For this review, use the dimensioned drawing (mm, ordinates from the lowest corner) and the shaded views. A direction names the side the tool comes from. Round coordinates to 2 decimals unless told otherwise and drop trailing zeros. Loops run counter-clockwise (first coordinate to the right, second up) from the corner with the lowest first, then second, coordinate; pieces in that order, holes last. Notation, with made-up numbers: (43.25, -31) - (65.25, -31) arc R25 cw to (65.25, 3) - close; hole circle Ø6 at (25, 1.5). An arc over 180 degrees is marked (long way). Use one line per item in the form item = value. Start each with the question number.
(1) For pin 1 (2 mm diameter, centred on y = 14, z = 6, fed in from -X); pin 2 (8 mm diameter, centred on y = 16.5, z = 3, fed in from +X); pin 3 (6 mm diameter, centred on x = 10.5, y = 9.5, fed in from +Z); pin 4 (4 mm diameter, centred on y = 16.5, z = 12, fed in from -X), all flat-tipped, find the tip position at first contact; note any pin that passes through.
(2) Wall thickness on probe 1 along Z at (x, y) = (17.5, 7.25); probe 2 along X at (y, z) = (6.75, 2.5); probe 3 along Y at (x, z) = (15.25, 12.5): over which ranges is each line inside the solid? List them lowest first. Write a range as [from, to].
(3) We need section C-C, the plane z = 2.5. Write out the cut boundary in (x, y).
(4) We need section A-A, the plane z = 6.5. Write out the cut boundary in (x, y) (1 decimal).
(5) The part is to be moulded in two halves that separate along X. For the marked faces 3, 4, 5 and 6, say which applies: released by +X, released by -X, zero draft, split by the parting line, or undercut.
(6) Machinability: for the marked faces 1 and 2, which of the approach directions +Z, -Z, +X, -X, +Y, -Y give a long, thin tool a straight path to every point of the face, cutting with its end or side? Answer none if there is none.
(7) We need section B-B, the plane y = 9.5. Write out the cut boundary in (x, z), then the cut area to 3 significant figures.
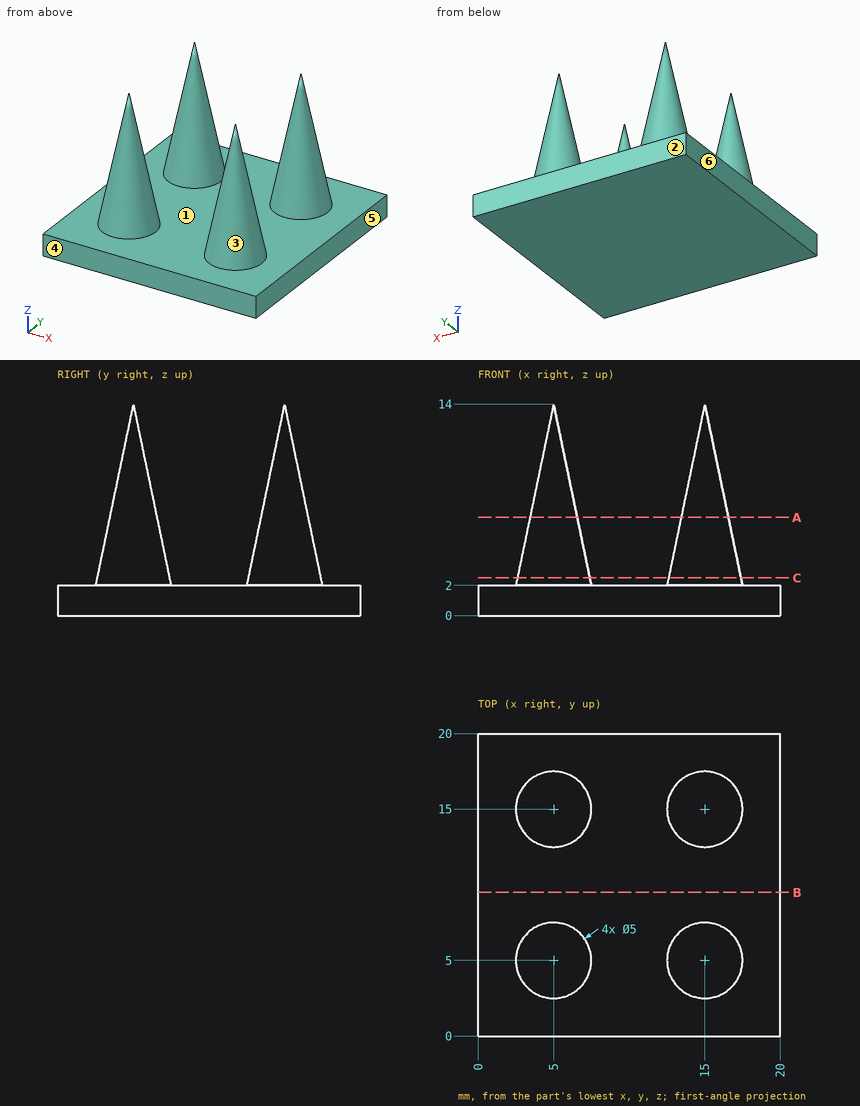
Data:
q1.pin_1 = 3.21
q1.pin_2 = 20
q1.pin_3 = 2
q1.pin_4 = 4.29
q2.probe_1 = [0, 2]
q2.probe_2 = [3.36, 6.64], [13.36, 16.64]
q2.probe_3 = [4.81, 5.19], [14.81, 15.19]
q3.outline = circle Ø4.79 at (5, 5); circle Ø4.79 at (5, 15); circle Ø4.79 at (15, 5); circle Ø4.79 at (15, 15)
q4.outline = circle Ø3.1 at (5, 5); circle Ø3.1 at (5, 15); circle Ø3.1 at (15, 5); circle Ø3.1 at (15, 15)
q5.face_3 = undercut
q5.face_4 = zero draft
q5.face_5 = released by +X
q5.face_6 = released by -X
q6.face_1 = +Z
q6.face_2 = +Z, -Z, +X, -X, +Y
q7.outline = (0, 0) - (20, 0) - (20, 2) - (0, 2) - close
q7.area = 40.0 mm^2
